from build123d import *

# Parameters (mm, degrees)
SKETCH1_R           = 25
BOSS_EXTRUDE1_DEPTH = 24
CUT_EXTRUDE3_START  = -2
CUT_EXTRUDE3_DEPTH  = 45.731721238
CIRPATTERN1_COUNT   = 6
CUT_EXTRUDE4_DEPTH  = 24
CIRPATTERN5_COUNT   = 6
CUT_EXTRUDE5_DEPTH  = 18
SKETCH6_R           = 1.9
CUT_EXTRUDE6_DEPTH  = 18


with BuildPart() as part:
    # Sketch1 → Boss-Extrude1 (new body)
    with BuildSketch(Plane(origin=(0, 0, 0), x_dir=(1, 0, 0), z_dir=(0, 1, 0))):
        with Locations(Location((0, 0, 0), (0, 0, 270))):
            Circle(SKETCH1_R)
    extrude(amount=BOSS_EXTRUDE1_DEPTH)

    # Sketch2 → Cut-Extrude3 (cut)
    with BuildSketch(Plane(origin=(0, 0, 0), x_dir=(1, 0, 0), z_dir=(0, 1, 0)).offset(CUT_EXTRUDE3_START)):
        with BuildLine():
            Line((-3, 24.819347292), (-4, 20.615528128))
            ThreePointArc((-4, 20.615528128), (0, 21), (4, 20.615528128))
            Line((4, 20.615528128), (3, 24.819347292))
            ThreePointArc((3, 24.819347292), (0, 25), (-3, 24.819347292))
        make_face()
    cut_extrude3 = extrude(amount=CUT_EXTRUDE3_DEPTH, mode=Mode.SUBTRACT)

    # CirPattern1: Cut-Extrude3 ×6 about axis
    cirpattern1_axis = Axis((0, 0, 0), (0, 1, 0))
    for i in range(1, CIRPATTERN1_COUNT):
        add(cut_extrude3.rotate(cirpattern1_axis, i * 360 / CIRPATTERN1_COUNT), mode=Mode.SUBTRACT)

    # Sketch3 → Cut-Extrude4 (cut)
    with BuildSketch(Plane(origin=(0, 0, 0), x_dir=(1, 0, 0), z_dir=(0, 1, 0))):
        with BuildLine():
            ThreePointArc((7.065480282, 7.767173771), (8.051747799, 7.376947701), (9.04955872, 7.736632793))
            Line((9.04955872, 7.736632793), (12.107901914, 10.351266166))
            ThreePointArc((12.107901914, 10.351266166), (12.632451903, 11.444743237), (12.176913221, 12.568722465))
            ThreePointArc((12.176913221, 12.568722465), (8.75, 15.155444566), (4.796376338, 16.829877422))
            ThreePointArc((4.796376338, 16.829877422), (3.595212432, 16.662395879), (2.910508504, 15.661383727))
            Line((2.910508504, 15.661383727), (2.175341178, 11.705464141))
            ThreePointArc((2.175341178, 11.705464141), (2.362750212, 10.661491989), (3.19382966, 10.0024723))
            ThreePointArc((3.19382966, 10.0024723), (5.25, 9.09326674), (7.065480282, 7.767173771))
        make_face()
    cut_extrude4 = extrude(amount=CUT_EXTRUDE4_DEPTH, mode=Mode.SUBTRACT)

    # CirPattern5: Cut-Extrude4 ×6 about axis
    cirpattern5_axis = Axis((-0.262257429, 0, 0.454243191), (0, 1, 0))
    for i in range(1, CIRPATTERN5_COUNT):
        add(cut_extrude4.rotate(cirpattern5_axis, i * 360 / CIRPATTERN5_COUNT), mode=Mode.SUBTRACT)

    # Sketch5 → Cut-Extrude5 (cut)
    with BuildSketch(Plane(origin=(0, 24, 0), x_dir=(1, 0, 0), z_dir=(0, 1, 0))):
        Polygon((0, 6.92820323), (-6, 3.464101615), (-6, -3.464101615), (0, -6.92820323), (6, -3.464101615), (6, 3.464101615), align=None)
    extrude(amount=-CUT_EXTRUDE5_DEPTH, mode=Mode.SUBTRACT)

    # Sketch6 → Cut-Extrude6 (cut)
    with BuildSketch(Plane(origin=(0, 6, 0), x_dir=(1, 0, 0), z_dir=(0, 1, 0))):
        with Locations(Location((0, 0, 0), (0, 0, 270))):
            Circle(SKETCH6_R)
    extrude(amount=-CUT_EXTRUDE6_DEPTH, mode=Mode.SUBTRACT)


solid = part.part
For this review, take the finished solid that the model builds, in its own axes (mm). A direction names the side the tool comes from. Round coordinates to 2 decimals unless told otherwise and drop trailing zeros. Loops run counter-clockwise (first coordinate to the right, second up) from the corner with the lowest first, then second, coordinate; pieces in that order, holes last. Notation, with made-up numbers: (-36.5, -27.5) - (-11.5, -27.5) arc R21 cw to (-11.5, -2.5) - close; hole circle Ø7 at (-34, 43). An arc over 180 degrees is marked (long way). Use one line per item in the form item = value.
Item 1: Consider section A-A on z = 0. Write out the cut boundary in (x, y), then the cut area to 3 significant figures.
Answers:
outline = (-25, 0) - (-18.28, 0) - (-18.28, 24) - (-25, 24) - close; (-11.28, 0) - (-1.9, 0) - (-1.9, 6) - (-6, 6) - (-6, 24) - (-11.28, 24) - close; (1.9, 0) - (10.75, 0) - (10.75, 24) - (6, 24) - (6, 6) - (1.9, 6) - close; (17.76, 0) - (25, 0) - (25, 24) - (17.76, 24) - close
area = 625 mm^2
Item 2: Consider section D-D on x = -21. Write out the cut boundary in (y, z), then the cut area to 3 significant figures.
Answers:
outline = (0, -7.93) - (24, -7.93) - (24, 7.93) - (0, 7.93) - close
area = 380 mm^2
Item 3: Mouldability with a two-part tool opening along X and no side actions: class faces 4 (the cylindrical face through (-12.38, 11.83, -21.72)), 5 (the cylindrical face through (12.633, 11.832, 12.371)), 6 (the cylindrical face through (12.62, 11.83, -21.58)), 7 (the cylindrical face through (18.158, 11.832, -10.549)) as +X half, -X half, draft (parallel to the pull), parting line (faces both ways), or undercut.
Answers:
face_4 = -X half
face_5 = undercut
face_6 = +X half
face_7 = undercut
Item 4: Tool access review of faces 1 (the cylindrical face through (5.277, 11.832, 9.986)), 2 (the flat face through (-3.042, 15.126, 5.172)), 3 (the cylindrical face through (-12.62, 11.83, 21.58)): name each direction out of +Z, -Z, +X, -X, +Y, -Y from which nothing blocks a thin tool from reaching the whole face with its end or side.
Answers:
face_1 = +Y, -Y
face_2 = +Y
face_3 = +Z, -X, +Y, -Y
Item 5: For line 1 (X direction, y = 2.7, z = 0); line 2 (X direction, y = 17.5, z = -7); line 3 (Z direction, x = -12.5, y = 5.25), list the stretches that pass through material, from the lowest coordinate up.
Answers:
line_1 = -25 to -18.28, -11.28 to -1.9, 1.9 to 10.75, 17.76 to 25
line_2 = -24 to -20.02, -19.8 to 19.8, 20.02 to 24
line_3 = -21.65 to -12.76, -10.24 to -3.69, 4.6 to 11.15, 13.67 to 21.65
Item 6: Consider section B-B on y = 3. State how many separate pieces and enclosed holes the cut face has, then the cut area to 3 significant figures.
Answers:
separate_pieces = 1
enclosed_holes = 7
area = 1,400 mm^2
Item 7: Clearance check with flat-ended pins moving along their axes: P1, Ø6, axis at x = 0, z = 0, coming from the +Y side; P2, Ø2, axis at y = 20.5, z = -16.5, coming from the +X side; P3, Ø2, axis at y = 10.5, z = 1.5, coming from the -X side (3 decimals). State where each tip first meets the part, or that it passes through.
Answers:
P1 = 6
P2 = 19.62
P3 = -24.995
